Autodesk Fusion 360 part; units mm, degrees
sketch "Sketch1" plane through (0, 0, 0) normal (0, 0, 1) x (1, 0, 0)
  line L0 (0, 0) -> (15, 0)
  line L1 (15, 0) -> (15, 25)
  line L2 (15, 25) -> (0, 25)
  line L3 (0, 25) -> (0, 0)
  circle A0 centre (3, 22) radius 1.5
  circle A1 centre (12, 3) radius 1.5
  circle A2 centre (12, 22) radius 1.5
  circle A3 centre (3, 3) radius 1.5
  line L4 (7.5, 25) -> (7.5, 0) construction
  line L5 (7.5, 12.5) -> (11.5, 12.5) construction
  circle A4 centre (11.5, 12.5) radius 2.5
  dimension "d11" = 15
  dimension "d12" = 25
  dimension "d13" = 3
  dimension "d14" = 3
  dimension "d15" = 3
  dimension "d16" = 3
  dimension "d17" = 3
  dimension "d18" = 3
  dimension "d19" = 3
  dimension "d20" = 3
  dimension "d21" = 3
  dimension "d22" = 3
  dimension "d23" = 3
  dimension "d24" = 3
  dimension "d27" = 4
  dimension "d28" = 5
extrude "Extrude1" add sketch "Sketch1" along normal blind 3
sketch "Sketch2" plane through (0, 0, 3) normal (0, 0, 1) x (-1, 0, 0)
  circle A0 centre (-12, -22) radius 1.5
  circle A1 centre (-12, -3) radius 1.5
  circle A2 centre (-3, -22) radius 1.5
  circle A3 centre (-3, -3) radius 1.5
  circle A4 centre (-11.5, -12.5) radius 2.5
  line L0 (0, -25) -> (0, 0)
  line L1 (0, 0) -> (-15, 0)
  line L2 (-15, 0) -> (-15, -25)
  line L3 (-15, -25) -> (0, -25)
  circle A5 centre (-3, -22) radius 1.5
  circle A6 centre (-12, -22) radius 1.5
  circle A7 centre (-12, -3) radius 1.5
  circle A8 centre (-3, -3) radius 1.5
  line L4 (-7.5, -25) -> (-7.5, 0) construction
  line L5 (0, -12.5) -> (-15, -12.5) construction
  line L6 (-11.5, -16.5) -> (-11.5, -8.5)
  line L7 (-3.5, -8.5) -> (-3.5, -16.5)
  arc A9 (-11.5, -16.5) -> (-3.5, -16.5) centre (-7.5, -16.5) ccw
  arc A10 (-3.5, -8.5) -> (-11.5, -8.5) centre (-7.5, -8.5) ccw
  line L8 (-11.5, -12.5) -> (-3.5, -12.5) construction
  arc A11 (-11.5, -11) -> (-11.5, -14) centre (-11.5, -12.5) ccw
  circle A12 centre (-7.5, -8.5) radius 2
  dimension "d31" = 3
  dimension "d32" = 3
  dimension "d33" = 3
  dimension "d34" = 3
  dimension "d35" = 8
  dimension "d36" = 8
  dimension "d37" = 8
  dimension "d39" = 3
  dimension "d40" = 4
extrude "Extrude2" add sketch "Sketch2" along normal blind 3 contours A4 L6 A11 | L0 L1 L2 L3
extrude "Extrude3" cut sketch "Sketch2" against normal blind 1.5 contours A12
fillet "Fillet1" radius 1 4 edges at (15, 0, 3) (0, 0, 3) (0, 25, 3) (15, 25, 3)
sketch "Sketch3" plane through (0, 0, 0) normal (-1, 0, 0) x (0, -1, 0)
  line L0 (-24, 6) -> (-24, 0)
  line L1 (-24, 0) -> (-1, 0)
  line L2 (-1, 0) -> (-1, 6)
  line L3 (-1, 6) -> (-24, 6)
  line L4 (-25, 0) -> (-25, 6)
  line L5 (0, 0) -> (0, 6)
  line L6 (-25, 3) -> (0, 3) construction
  line L7 (-12.5, 6) -> (-12.5, 0) construction
  circle A0 centre (-12.5, 3) radius 2.5
  circle A1 centre (-12.5, 3) radius 1.5
  point P0 (-12.5, 0)
  dimension "d50" = 5
  dimension "d51" = 3
extrude "Extrude4" cut sketch "Sketch3" against normal blind 1.5 contours A0
extrude "Extrude5" cut sketch "Sketch3" against normal blind 3 contours A1
hole "Hole1" at (3, 12.5, 3) direction (1, 0, 0) diameter 3 depth 0.1 tip angle 118
equation "outer_filet_radius = 1 mm"
equation "mount_hole_diameter = 3 mm"
equation "mount_hole_length_inset = 3 mm"
equation "mount_hole_width_inset = 3 mm"
equation "bottom_thru_hole_diameter = 5 mm"
equation "bottom_plate_depth = 3 mm"
equation "bottom_plate_partial_hole_radius = 4 mm"
equation "bottom_plate_partial_hole_depth = 4.5 mm"
equation "width = 15 mm"
equation "length = 25 mm"
equation "d11 = width"
equation "d12 = length"
equation "d13 = mount_hole_diameter"
equation "d14 = mount_hole_diameter"
equation "d15 = mount_hole_diameter"
equation "d16 = mount_hole_diameter"
equation "d17 = mount_hole_width_inset"
equation "d18 = mount_hole_width_inset"
equation "d19 = mount_hole_width_inset"
equation "d20 = mount_hole_width_inset"
equation "d21 = mount_hole_length_inset"
equation "d22 = mount_hole_length_inset"
equation "d23 = mount_hole_length_inset"
equation "d24 = mount_hole_length_inset"
equation "slot_radius = 4 mm"
equation "slot_length = 16 mm"
equation "d27 = slot_radius"
equation "d28 = bottom_thru_hole_diameter"
equation "d29 = bottom_plate_depth"
equation "d31 = mount_hole_diameter"
equation "d32 = mount_hole_diameter"
equation "d33 = mount_hole_diameter"
equation "d34 = mount_hole_diameter"
equation "d35 = slot_radius * 2"
equation "d36 = slot_radius * 2"
equation "d37 = slot_length - ( slot_radius * 2 )"
equation "slotted_circle_diameter = 3 mm"
equation "d39 = slotted_circle_diameter"
equation "d40 = bottom_plate_partial_hole_radius"
equation "top_plate_thickness = 3 mm"
equation "d42 = top_plate_thickness"
equation "d44 = top_plate_thickness - bottom_plate_partial_hole_depth"
equation "d47 = outer_filet_radius"
equation "outer_side_hole_diameter = 5 mm"
equation "inner_side_hole_diameter = 3 mm"
equation "d50 = outer_side_hole_diameter"
equation "d51 = inner_side_hole_diameter"
equation "outer_side_hole_depth = 1.5 mm"
equation "inner_side_hole_depth = 3 mm"
Here's how the part is built. I have some questions about the finished solid (model axes, mm). A direction names the side the tool comes from. Give positions to 0.01 mm unless a question says otherwise; leave off trailing zeros. Order: outer loops, then holes, each group sorted by start corner. A loop starts at its lowest first (then second) coordinate and runs counter-clockwise, first axis right, second up. Notation, with made-up numbers: (52, 48) -> (63, 48) arc R20 cw to (63, 74) -> close; hole circle Ø11 at (45, -6). An arc over 180 degrees is marked (long way). Use CSV: the item, a comma, the result in double quotes. Start each with the question number.
Item 1: Suppose I cut it at D-D (y = 8). List the corners of the cut face in (x, z) for me, and give its area (3 significant figures).
Item 2: Suppose I cut it at C-C (y = 2.25). List the corners of the cut face in (x, z) for me, and give its area (3 significant figures).
Item 3: If I drill on probe 1 along X at (y, z) = (22, 3.95); probe 2 along Z at (x, y) = (1.1, 12.5); probe 3 along X at (y, z) = (10.75, 4.45), over which ranges is the centre line in solid material (lowest first)? Write a range as [from, to].
Item 4: On a 3-axis mill with a long thin cutter (end or side, diameter ignored), from which of +Z, -Z, +X, -X, +Y, -Y can I reach the whole of each face in a straight line? I mean faces 1 (the flat face through (1.5, 11, 2)), 2 (the cylindrical face through (7.6, 4.5, 4.5)), 3 (the cylindrical face through (13, 12.5, 4.5)), 4 (the cylindrical face through (10.96, 14.94, 1.48)), 5 (the flat face through (15, 12, 3)). Say none if no direction works.
Item 5: I'm going to push flat-ended pins straight in: P1, Ø2.5, axis at y = 13.5, z = 3.5, coming from the -X side; P2, Ø1.2, axis at x = 13, y = 12, coming from the -Z side; P3, Ø4, axis at x = 7.5, y = 12, coming from the +Z side. Where does each tip first touch, or does it pass through?
Item 6: Suppose I cut it at B-B (z = 5.05). List the corners of the cut face in (x, y) for me.
Item 7: Thinking about a two-plate mould opening in Y: for faces 6 (the cylindrical face through (1, 15, 3)), 7 (the flat face through (7, 0, 3)), 8 (the flat face through (0, 15.2, 3)), which applies, pulls with the +Y half, pulls with the -Y half, needs draft (parallel to the pull), parting line crosses it, or undercut?
Answer block:
1,outline,"(0, 0) -> (15, 0) -> (15, 6) -> (11.47, 6) -> (11.47, 3) -> (9.44, 3) -> (9.44, 1.5) -> (5.56, 1.5) -> (5.56, 3) -> (3.53, 3) -> (3.53, 6) -> (0, 6) -> close"
1,area,"60.4 mm^2"
2,outline,"(0, 0) -> (1.7, 0) -> (1.7, 6) -> (0, 6) -> close; (4.3, 0) -> (10.7, 0) -> (10.7, 6) -> (4.3, 6) -> close; (13.3, 0) -> (15, 0) -> (15, 6) -> (13.3, 6) -> close"
2,area,"58.8 mm^2"
3,probe 1,"x = [0, 1.5], [4.5, 10.5], [13.5, 15]"
3,probe 2,"z = [0, 0.5], [5.5, 6]"
3,probe 3,"x = [1.5, 3.5], [11.5, 15]"
4,face 1,"-X"
4,face 2,"+Z"
4,face 3,"+Z, -Z"
4,face 4,"-Z"
4,face 5,"+Z, -Z, +X, +Y, -Y"
5,P1,"stops at x = 1.5"
5,P2,"stops at z = 3"
5,P3,"stops at z = 3"
6,outline,"(0, 1) arc R1 ccw to (1, 0) -> (14, 0) arc R1 ccw to (15, 1) -> (15, 24) arc R1 ccw to (14, 25) -> (1, 25) arc R1 ccw to (0, 24) -> (0, 13.93) -> (1.5, 13.93) -> (1.5, 11.07) -> (0, 11.07) -> close; hole circle Ø3 at (3, 3); hole circle Ø3 at (3, 22); hole (3.5, 8.5) arc R4 ccw to (11.5, 8.5) -> (11.5, 11) arc R1.5 ccw to (11.5, 14) -> (11.5, 16.5) arc R4 ccw to (3.5, 16.5) -> close; hole circle Ø3 at (12, 3); hole circle Ø3 at (12, 22)"
7,face 6,"undercut"
7,face 7,"pulls with the -Y half"
7,face 8,"needs draft"
